The model under review builds one solid part; all positions refer to its coordinate system, in mm. Face numbers are marked on the shaded views. A direction names the side the tool comes from. Round coordinates to 2 decimals unless told otherwise and drop trailing zeros. Write each loop counter-clockwise with the first axis right and the second up, starting at its lowest first coordinate (ties: lowest second). Pieces come first, ordered by that corner, then holes. Notation, with made-up numbers: (85.25, 25) - (132.25, 25) arc R16 ccw to (132.25, 38) - close; hole circle Ø9 at (59.5, -37). An arc over 180 degrees is marked (long way). Return JSON: item names as keys, results as strings.
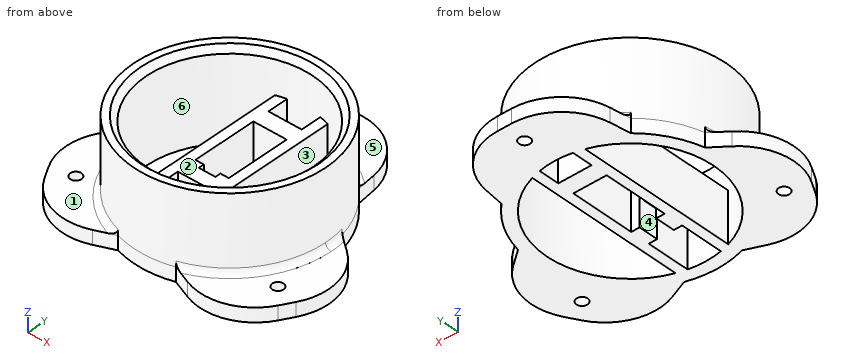
from build123d import *

# Parameters (mm, degrees)
F0_R         = 2
F0_R_2       = 30
F1_DEPTH     = 5
F2_R         = 34.5
F2_R_2       = 30
F3_DEPTH     = 27
F5_DEPTH     = 18
F6_SIZE      = 2
F7_T4_ANGLE  = 101.4429805126
F7_T10_ANGLE = 101.4429805126
F7_T16_ANGLE = 20.718590379
F7_T21_ANGLE = 80.7206862136
F8_W         = 6
F8_H         = 5
F9_DEPTH     = 10


# Not quite as in the source:
# - a fillet or chamfer that OpenCascade refuses, or shapes differently, is made with other operations: its cross-section is extruded or revolved along the edge and cut away or added


with BuildPart() as f1:
    # F0 (on Top) → F1 (new body)
    with BuildSketch(Plane.XY):
        with BuildLine():
            Line((2.4892725641, 50), (-2.4892725641, 50))
            ThreePointArc((-2.4892725641, 50), (-15.663935341, 45.0475333764), (-22.31389035, 32.6428260715))
            Line((-22.31389035, 32.6428260715), (-23.2700083459, 25.4707030052))
            ThreePointArc((-23.2700083459, 25.4707030052), (-29.8778764306, 17.25), (-33.6932800277, 7.4170668712))
            Line((-33.6932800277, 7.4170668712), (-39.4264618042, 3.0029828646))
            ThreePointArc((-39.4264618042, 3.0029828646), (-46.8442759523, -8.9584007597), (-44.5459064713, -22.8442267226))
            Line((-44.5459064713, -22.8442267226), (-42.0566339072, -27.1557732774))
            ThreePointArc((-42.0566339072, -27.1557732774), (-31.1803406113, -36.0891326167), (-17.1125714543, -35.6458089361))
            Line((-17.1125714543, -35.6458089361), (-10.4232716818, -32.8877698765))
            ThreePointArc((-10.4232716818, -32.8877698765), (0, -34.5), (10.4232716818, -32.8877698765))
            Line((10.4232716818, -32.8877698765), (17.1125714543, -35.6458089361))
            ThreePointArc((17.1125714543, -35.6458089361), (31.1803406113, -36.0891326167), (42.0566339072, -27.1557732774))
            Line((42.0566339072, -27.1557732774), (44.5459064713, -22.8442267226))
            ThreePointArc((44.5459064713, -22.8442267226), (46.8442759523, -8.9584007597), (39.4264618042, 3.0029828646))
            Line((39.4264618042, 3.0029828646), (33.6932800277, 7.4170668712))
            ThreePointArc((33.6932800277, 7.4170668712), (29.8778764306, 17.25), (23.2700083459, 25.4707030052))
            Line((23.2700083459, 25.4707030052), (22.31389035, 32.6428260715))
            ThreePointArc((22.31389035, 32.6428260715), (15.663935341, 45.0475333764), (2.4892725641, 50))
        make_face()
        with Locations((-36.3730669589, -21)):
            Circle(F0_R, mode=Mode.SUBTRACT)
        with Locations((36.3730669589, -21)):
            Circle(F0_R, mode=Mode.SUBTRACT)
        Circle(F0_R_2, mode=Mode.SUBTRACT)
        with Locations((0, 42)):
            Circle(F0_R, mode=Mode.SUBTRACT)
    extrude(amount=F1_DEPTH)

    # F2 (on face) → F3 (join)
    with BuildSketch(Plane.XY.offset(5)):
        Circle(F2_R)
        Circle(F2_R_2, mode=Mode.SUBTRACT)
    extrude(amount=F3_DEPTH)

    # F4 (on Top) → F5 (join)
    with BuildSketch(Plane.XY):
        with BuildLine():
            Line((9.5, 0), (9.5, 28.4561065503))
            ThreePointArc((9.5, 28.4561065503), (7.7641711286, 28.9778820255), (6, 29.3938769134))
            Line((6, 29.3938769134), (6, 22))
            Line((6, 22), (0, 22))
            Line((0, 22), (-6, 22))
            Line((-6, 22), (-6, 29.3938769134))
            ThreePointArc((-6, 29.3938769134), (-7.7641711286, 28.9778820255), (-9.5, 28.4561065503))
            Line((-9.5, 28.4561065503), (-9.5, 0))
            Line((-9.5, 0), (-9.5, -28.4561065503))
            ThreePointArc((-9.5, -28.4561065503), (-7.7641711286, -28.9778820255), (-6, -29.3938769134))
            Line((-6, -29.3938769134), (-6, -14))
            Line((-6, -14), (-6, -9))
            Line((-6, -9), (-6, -7))
            Line((-6, -7), (-6, 16))
            Line((-6, 16), (0, 16))
            Line((0, 16), (6, 16))
            Line((6, 16), (6, -7))
            Line((6, -7), (6, -9))
            Line((6, -9), (6, -14))
            Line((6, -14), (6, -29.3938769134))
            ThreePointArc((6, -29.3938769134), (7.7641711286, -28.9778820255), (9.5, -28.4561065503))
            Line((9.5, -28.4561065503), (9.5, 0))
        make_face()
        Polygon((0, -14), (6, -14), (6, -9), (6, -7), (3, -7), (3, -9), (-3, -9), (-3, -7), (-6, -7), (-6, -9), (-6, -14), align=None)
    extrude(amount=F5_DEPTH)

    # F6
    f6_edges = [f1.edges().sort_by_distance(p)[0] for p in [
        (-30, 0, 32),
    ]]
    chamfer(f6_edges, length=F6_SIZE)

    # F7: fillet of radius 2 on 3 edges, made by hand


with BuildPart() as f7_tool2:
    # F7_s3 → F7_t4 (revolve)
    with BuildSketch(Plane(origin=(0, 0, 0), x_dir=(0, 0, 1), z_dir=(0.3538256813, 0.9353113852, 0))):
        with BuildLine():
            ThreePointArc((7, -34.5), (5.5857864376, -35.0857864376), (5, -36.5))
            Line((5, -36.5), (5, -34.5))
            Line((5, -34.5), (7, -34.5))
        make_face()
    revolve(axis=Axis((0, 0, 5), (0, 0, 1)), revolution_arc=F7_T4_ANGLE)

    split(bisect_by=Plane(origin=(-16.1247319925, 20.9434209841, 0), x_dir=(0, 0, 1), z_dir=(0.6100531704, -0.7923604794, 0)), keep=Keep.TOP)

    split(bisect_by=Plane(origin=(10.0751686181, -24.4361380268, 0), x_dir=(0, 0, 1), z_dir=(-0.3811777189, 0.9245017829, 0)), keep=Keep.TOP)


with BuildPart() as f1_1:
    add(f1.part)

    # F7_t1: union F7_tool2
    add(f7_tool2.part)


with BuildPart() as f7_tool8:
    # F7_s9 → F7_t10 (revolve)
    with BuildSketch(Plane(origin=(0, 0, 0), x_dir=(0, 0, 1), z_dir=(0.6330905794, -0.7740777211, 0))):
        with BuildLine():
            ThreePointArc((7, -34.5), (5.5857864376, -35.0857864376), (5, -36.5))
            Line((5, -36.5), (5, -34.5))
            Line((5, -34.5), (7, -34.5))
        make_face()
    revolve(axis=Axis((0, 0, 5), (0, 0, 1)), revolution_arc=F7_T10_ANGLE)

    split(bisect_by=Plane(origin=(-26.1999006106, 3.4927170427, 0), x_dir=(0, 0, 1), z_dir=(0.9912308893, -0.1321413036, 0)), keep=Keep.TOP)

    split(bisect_by=Plane(origin=(26.1999006106, 3.4927170427, 0), x_dir=(0, 0, 1), z_dir=(-0.9912308893, -0.1321413036, 0)), keep=Keep.TOP)


with BuildPart() as f1_2:
    add(f1_1.part)

    # F7_t7: union F7_tool8
    add(f7_tool8.part)


with BuildPart() as f7_tool14:
    # F7_s15 → F7_t16 (revolve)
    with BuildSketch(Plane.XZ):
        with BuildLine():
            ThreePointArc((34.5, 7), (35.0857864376, 5.5857864376), (36.5, 5))
            Line((36.5, 5), (34.5, 5))
            Line((34.5, 5), (34.5, 7))
        make_face()
    revolve(axis=Axis((0, 0, 5), (0, 0, 1)), revolution_arc=F7_T16_ANGLE)

    split(bisect_by=Plane(origin=(16.1247319925, 20.9434209841, 0), x_dir=(0, 0, 1), z_dir=(-0.6100531704, -0.7923604794, 0)), keep=Keep.TOP)


with BuildPart() as f1_3:
    add(f1_2.part)

    # F7_t13: union F7_tool14
    add(f7_tool14.part)


with BuildPart() as f7_tool19:
    # F7_s20 → F7_t21 (revolve)
    with BuildSketch(Plane(origin=(0, 0, 0), x_dir=(0, 0, 1), z_dir=(-0.9869139979, -0.1612475137, 0))):
        with BuildLine():
            ThreePointArc((7, -34.5), (5.5857864376, -35.0857864376), (5, -36.5))
            Line((5, -36.5), (5, -34.5))
            Line((5, -34.5), (7, -34.5))
        make_face()
    revolve(axis=Axis((0, 0, 5), (0, 0, 1)), revolution_arc=F7_T21_ANGLE)

    split(bisect_by=Plane(origin=(-10.0751686181, -24.4361380268, 0), x_dir=(0, 0, 1), z_dir=(0.3811777189, 0.9245017829, 0)), keep=Keep.TOP)


with BuildPart() as f1_4:
    add(f1_3.part)

    # F7_t18: union F7_tool19
    add(f7_tool19.part)

    # F8 (on face) → F9 (cut)
    with BuildSketch(Plane(origin=(0, 0, 0), x_dir=(1, 0, 0), z_dir=(0, 0, -1))):
        with Locations((0, 11.5)):
            Rectangle(F8_W, F8_H)
    extrude(amount=-F9_DEPTH, mode=Mode.SUBTRACT)


solid = f1_4.part
(1) Add section A-A (z = 12). Write out the cut boundary in (x, y).
Filled in:
{"outline": "circle Ø69 at (0, 0); hole (-9.5, -28.46) - (-9.5, 28.46) arc R30 ccw to start; hole (-6, -29.39) arc R30 ccw to (6, -29.39) - (6, -14) - (-6, -14) - close; hole (-6, -7) - (-3, -7) - (-3, -9) - (3, -9) - (3, -7) - (6, -7) - (6, 16) - (-6, 16) - close; hole (-6, 22) - (6, 22) - (6, 29.39) arc R30 ccw to (-6, 29.39) - close; hole (9.5, -28.46) arc R30 ccw to (9.5, 28.46) - close"}
(2) Wall thickness on line 1 (X direction, y = 0, z = 13); line 2 (Y direction, x = 0, z = 2.35); line 3 (Y direction, x = 0, z = 10.5): over which ranges is each line inside the solid? List them lowest first.
Filled in:
{"line 1": "x = -34.5 to -30, -9.5 to -6, 6 to 9.5, 30 to 34.5", "line 2": "y = -34.5 to -30, 16 to 22, 30 to 40, 44 to 50", "line 3": "y = -34.5 to -30, -14 to -9, 16 to 22, 30 to 34.5"}
(3) Add section C-C (y = 42). Write out the cut boundary in (x, z), plus the area to 3 significant figures.
Filled in:
{"outline": "(-18.49, 0) - (-2, 0) - (-2, 5) - (-18.49, 5) - close; (2, 0) - (18.49, 0) - (18.49, 5) - (2, 5) - close", "area": "165 mm2"}
(4) Add section D-D (z = 3). Give the number of separate pieces and of enclosed holes in the cut face, plus the area to 3 significant figures.
Filled in:
{"separate pieces": "1", "enclosed holes": "7", "area": "3,340 mm2"}
(5) Mouldability with a two-part tool opening along Y and no side actions: class the marked faces 5 and 6 as released by +Y, released by -Y, zero draft, split by the parting line, or undercut.
Filled in:
{"face 5": "zero draft", "face 6": "undercut"}
(6) Clearance check with flat-ended pins moving along their axes: pin 1 Ø1 at (x, z) = (32, 18) entering from -Y; pin 2 Ø6 at (x, z) = (-17, 16.5) entering from +Y; pin 3 Ø4.5 at (y, z) = (-21, 13) entering from +X; pin 4 Ø6 at (y, z) = (39, 11.5) entering from +X. State where each tip first meets the part, or that it passes through.
Filled in:
{"pin 1": "stops at y = -14.07", "pin 2": "stops at y = 31.53", "pin 3": "stops at x = 28.96", "pin 4": "passes through"}
(7) Add section B-B (x = 0). Write out the cut boundary in (y, z), plus the area to 3 significant figures.
Filled in:
{"outline": "(-34.5, 0) - (-30, 0) - (-30, 30) - (-32, 32) - (-34.5, 32) - close; (-14, 10) - (-9, 10) - (-9, 18) - (-14, 18) - close; (16, 0) - (22, 0) - (22, 18) - (16, 18) - close; (30, 0) - (40, 0) - (40, 5) - (36.5, 5) arc R2 cw to (34.5, 7) - (34.5, 32) - (32, 32) - (30, 30) - close; (44, 0) - (50, 0) - (50, 5) - (44, 5) - close", "area": "490 mm2"}
(8) For the marked faces 1, 2, 3 and 4, list the 3-axis set-ups (+Z, -Z, +X, -X, +Y, -Y) from which the entire face can be reached by the end or side of a thin tool; tool diameter is ignored.
Filled in:
{"face 1": "+Z, -X, -Y", "face 2": "+Z", "face 3": "+Z, -Z", "face 4": "-Z"}
